Check sheet for the modelled part. Datum: model origin and axes. Units: mm. A direction names the side the tool comes from. Coordinates: 2 decimals unless noted, no trailing zeros. Loops run counter-clockwise (first coordinate to the right, second up) from the corner with the lowest first, then second, coordinate; pieces in that order, holes last.
```python
from build123d import *

# Parameters (mm, degrees)
F0_R      = 24.511
F1_DEPTH  = 24.4348
F2_R      = 3.4925
F3_DEPTH  = 18.415
F4_R      = 6.0071
F5_DEPTH  = 1.778
F6_SIZE   = 1.27
F7_R      = 1.5367
F8_DEPTH  = 12.7
F9_R      = 2.1336
F10_DEPTH = 0.9652
F11_R     = 2.032


with BuildPart() as f1:
    # F0 (on Front) → F1 (new body)
    with BuildSketch(Plane.XZ):
        Circle(F0_R)
    extrude(amount=F1_DEPTH)

    # F2 (on face) → F3 (join)
    with BuildSketch(Plane(origin=(0, 0, 0), x_dir=(-1, 0, 0), z_dir=(0, 1, 0))):
        with Locations((0, -11.7475)):
            Circle(F2_R)
    extrude(amount=F3_DEPTH)

    # F4 (on face) → F5 (join)
    with BuildSketch(Plane(origin=(0, 0, 0), x_dir=(-1, 0, 0), z_dir=(0, 1, 0))):
        with Locations((0, -11.7475)):
            Circle(F4_R)
    extrude(amount=F5_DEPTH)

    # F6
    f6_edges = [f1.edges().sort_by_distance(p)[0] for p in [
        (3.4925, 18.415, -11.7475),
    ]]
    chamfer(f6_edges, length=F6_SIZE)

    # F7 (on Right) → F8 (cut, symmetric)
    with BuildSketch(Plane.YZ):
        with Locations((14.605, -11.811)):
            Circle(F7_R)
    extrude(amount=F8_DEPTH, both=True, mode=Mode.SUBTRACT)

    # F9 (on face) → F10 (join)
    with BuildSketch(Plane(origin=(0, 0, 0), x_dir=(-1, 0, 0), z_dir=(0, 1, 0))):
        with BuildLine():
            ThreePointArc((21.7190408618, 11.3610028186), (24.0387512815, 4.788272948), (24.414607206, -2.1716528208))
            Line((24.414607206, -2.1716528208), (32.2426542084, -1.1577105466))
            Line((32.2426542084, -1.1577105466), (30.4742566429, 12.4950383448))
            Line((30.4742566429, 12.4950383448), (21.7190408618, 11.3610028186))
        make_face()
        with Locations((28.575, 1.2954)):
            Circle(F9_R, mode=Mode.SUBTRACT)
        with Locations((27.559, 7.5635930411)):
            Circle(F9_R, mode=Mode.SUBTRACT)
        with BuildLine():
            ThreePointArc((-24.414607206, -2.1716528208), (-24.044022755, 4.7617319075), (-21.7440723776, 11.3130207036))
            Line((-21.7440723776, 11.3130207036), (-30.4807820952, 12.4446591976))
            Line((-30.4807820952, 12.4446591976), (-32.2426542084, -1.1577105466))
            Line((-32.2426542084, -1.1577105466), (-24.414607206, -2.1716528208))
        make_face()
        with Locations((-28.575, 1.2954)):
            Circle(F9_R, mode=Mode.SUBTRACT)
        with Locations((-27.559, 7.5635930411)):
            Circle(F9_R, mode=Mode.SUBTRACT)
    extrude(amount=-F10_DEPTH)

    # F11
    f11_edges = [f1.edges().sort_by_distance(p)[0] for p in [
        (-24.511, -24.4348, 0),
    ]]
    fillet(f11_edges, radius=F11_R)


solid = f1.part
```
1) Set-up check for faces 4 (the cylindrical face through (0.78, 0.88, -5.79)), 5 (the cylindrical face through (23.38, -11.04, 7.36)), 6 (the cylindrical face through (-30.61, -0.48, 1.94)): record each of +Z, -Z, +X, -X, +Y, -Y from which the full face is reachable in a straight line by a thin tool's end or side.
Answer sheet:
face 4: +Y
face 5: -Y
face 6: +Y, -Y
2) Scan lines: line 1 (Y direction, x = 12, z = -7.5); line 2 (Z direction, x = -1.5, y = 15.5); line 3 (Z direction, x = -1, y = 14). Record each from-to range of solid material in increasing order.
Answer sheet:
line 1: y = -24.43 to 0
line 2: z = -14.9 to -13.06, -10.56 to -8.59
line 3: z = -15.09 to -13.22, -10.4 to -8.4
3) Mould release check, pull along Y, two halves, no side actions. Record for faces 1 (the flat face through (-3, 1.778, -14)), 2 (the cylindrical face through (0.05, 14.4, -10.29)), 3 (the cylindrical face through (-28.54, -0.48, 5.67)): +Y half, -Y half, draft (parallel to the pull), parting line (faces both ways), or undercut.
Answer sheet:
face 1: +Y half
face 2: undercut
face 3: draft
4) Section check A-A on z = 0. Enter the section's corners in (x, y), plus the area to 3 significant figures.
Answer sheet:
outline: (-32.09, -0.97) - (-30.27, -0.97) - (-30.27, 0) - (-32.09, 0) - close; (-26.88, -0.97) - (-24.51, -0.97) - (-24.51, -22.4) arc R2.03 ccw to (-22.48, -24.43) - (22.48, -24.43) arc R2.03 ccw to (24.51, -22.4) - (24.51, -0.97) - (26.88, -0.97) - (26.88, 0) - (-26.88, 0) - close; (30.27, -0.97) - (32.09, -0.97) - (32.09, 0) - (30.27, 0) - close
area: 1,200 mm2
5) Section check C-C on y = -6. Enter the section's corners in (x, z), plus the area to 3 significant figures.
Answer sheet:
outline: circle Ø49.02 at (0, 0)
area: 1,890 mm2
6) Section check D-D on y = 7.5. Enter the section's corners in (x, z) (1 decimal).
Answer sheet:
outline: circle Ø7 at (0, -11.7)
7) Depth check by flat-ended pin: pin 1 (4 mm diameter, centred on x = 28.58, z = 1.3, fed in from -Y); pin 2 (10 mm diameter, centred on x = -5.5, y = -11, fed in from +Z); pin 3 (5.5 mm diameter, centred on x = -26, z = 8.5, fed in from -Y); pin 4 (3.5 mm diameter, centred on x = 3, z = -14.5, fed in from +Y). Enter the tip coordinate at first touch or a pass-through.
Answer sheet:
pin 1: passes through
pin 2: stops at z = 24.51
pin 3: stops at y = -0.97
pin 4: stops at y = 18.32
8) Section check B-B on x = 0. Enter the section's corners in (y, z) (3 decimals).
Answer sheet:
outline: (-24.435, -22.479) arc R2.032 ccw to (-22.403, -24.511) - (0, -24.511) - (0, -17.755) - (1.778, -17.755) - (1.778, -15.24) - (17.145, -15.24) - (18.415, -13.97) - (18.415, -9.525) - (17.145, -8.255) - (1.778, -8.255) - (1.778, -5.74) - (0, -5.74) - (0, 24.511) - (-22.403, 24.511) arc R2.032 ccw to (-24.435, 22.479) - close; hole circle Ø3.073 at (14.605, -11.811)
